```python
from build123d import *

# Parameters (mm, degrees)
F1_DEPTH = 15


with BuildPart() as f1:
    # F0 (on Top) → F1 (new body)
    with BuildSketch(Plane.XY):
        with BuildLine():
            Line((550, 0), (0, 0))
            Line((0, 0), (0, -800))
            ThreePointArc((0, -800), (176.776695, -726.776695), (250, -550))
            Line((250, -550), (250, -300))
            ThreePointArc((250, -300), (264.644661, -264.644661), (300, -250))
            ThreePointArc((300, -250), (476.776695, -176.776695), (550, 0))
        make_face()
    extrude(amount=F1_DEPTH)


solid = f1.part
```
Source: CAD feature listing. Evaluate the final solid. Frame: model axes, mm. A direction names the side the tool comes from. Round coordinates to 2 decimals unless told otherwise and drop trailing zeros. Loops run counter-clockwise (first coordinate to the right, second up) from the corner with the lowest first, then second, coordinate; pieces in that order, holes last. Notation, with made-up numbers: M 65.5,43.25 L 90.5,43.25 A28 ccw 90.5,68.25 Z; hole C -14.5,50 d9. An arc over 180 degrees is marked long. Use a Markdown table: item, result. Add a question column.
1. Cut plane A-A, the plane y = -355. Output: boundary loops of the cut face in (x, z).
2. Cut plane C-C, the plane x = 176. Output: boundary loops of the cut face in (y, z).
3. Set-up query: faces 1 (the flat face through (250, -427, 7)), 2 (the flat face through (279, 0, 7)). Return all of +Z, -Z, +X, -X, +Y, -Y with unobstructed straight access to the full face (end or side cutting, diameter ignored); none if empty.
4. Contact query for flat-ended pins moving along their axis: pin 1 (6 mm diameter, centred on x = 226.5, y = -284, fed in from -Z); pin 2 (4 mm diameter, centred on y = -589.5, z = 8, fed in from +X); pin 3 (7.5 mm diameter, centred on y = -391.5, z = 4.5, fed in from +X); pin 4 (1.5 mm diameter, centred on y = -261.5, z = 12, fed in from +X). Output: stop coordinate, or through.
5. Cut plane B-B, the plane z = 5. Output: boundary loops of the cut face in (x, y), and give its area (3 significant figures).
6. Ray query, line 1 along X through (y, z) = (-532.5, 2); line 2 along X through (y, z) = (-627.5, 4.5); line 3 along Y through (x, z) = (353.5, 2). Return the intervals inside material, ascending. Write a range as [from, to].
Solution:
| question | item | result |
|---|---|---|
| 1 | outline | M 0,0 L 250,0 L 250,15 L 0,15 Z |
| 2 | outline | M -727.55,0 L 0,0 L 0,15 L -727.55,15 Z |
| 3 | face 1 | +Z, -Z, +X, -Y |
| 3 | face 2 | +Z, -Z, +X, -X, +Y |
| 4 | pin 1 | stops at z = 0 |
| 4 | pin 2 | stops at x = 247.17 |
| 4 | pin 3 | stops at x = 250 |
| 4 | pin 4 | stops at x = 269.03 |
| 5 | outline | M 0,-800 A250 ccw 250,-550 L 250,-300 A50 cw 300,-250 A250 ccw 550,0 L 0,0 Z |
| 5 | area | 249,000 mm2 |
| 6 | line 1 | x = [0, 250] |
| 6 | line 2 | x = [0, 237.68] |
| 6 | line 3 | y = [-244.21, 0] |
